from build123d import *

# Parameters (mm, degrees)
F1_DEPTH        = 25
F2_DEPTH        = 30
F3_W            = 11.9576826692
F3_H            = 39.7608936764
F4_DEPTH        = 40
F5_R            = 15.1725757167
F6_DEPTH        = 68.3238299022
F7_T1_DEPTH     = 111.9576826692
F7_T3_DEPTH     = 111.9576826692
F8_R            = 9
F10_D           = 8
F10_DEPTH       = 10
F10_CBORE_D     = 10
F10_CBORE_DEPTH = 5
F10_TIP         = 2.4034424761


# Not quite as in the source:
# - a fillet or chamfer that OpenCascade refuses, or shapes differently, is made with other operations: its cross-section is extruded or revolved along the edge and cut away or added


with BuildPart() as f1:
    # F0 (on Top) → F1 (new body)
    with BuildSketch(Plane.XY):
        with BuildLine():
            Line((8.5056748986, -46.3761053979), (13.5056748986, -46.3761053979))
            Line((13.5056748986, -46.3761053979), (13.5056748986, -23.932851851))
            ThreePointArc((13.5056748986, -23.932851851), (0, -10.4271769524), (-13.5056748986, -23.932851851))
            Line((-13.5056748986, -23.932851851), (-13.5056748986, -46.3761053979))
            Line((-13.5056748986, -46.3761053979), (-8.5056748986, -46.3761053979))
            Line((-8.5056748986, -46.3761053979), (-8.5056748986, -23.932851851))
            ThreePointArc((-8.5056748986, -23.932851851), (0, -15.4271769524), (8.5056748986, -23.932851851))
            Line((8.5056748986, -23.932851851), (8.5056748986, -46.3761053979))
        make_face()
    extrude(amount=F1_DEPTH)

    # F0 (on Top) → F2 (join)
    with BuildSketch(Plane.XY):
        with BuildLine():
            Line((34.1614149511, -46.3761053979), (34.1614149511, 46.3761053979))
            Line((34.1614149511, 46.3761053979), (-34.1614149511, 46.3761053979))
            Line((-34.1614149511, 46.3761053979), (-34.1614149511, -46.3761053979))
            Line((-34.1614149511, -46.3761053979), (-13.5056748986, -46.3761053979))
            Line((-13.5056748986, -46.3761053979), (-13.5056748986, -23.932851851))
            ThreePointArc((-13.5056748986, -23.932851851), (0, -10.4271769524), (13.5056748986, -23.932851851))
            Line((13.5056748986, -23.932851851), (13.5056748986, -46.3761053979))
            Line((13.5056748986, -46.3761053979), (34.1614149511, -46.3761053979))
        make_face()
    extrude(amount=F2_DEPTH)

    # F3 (on face) → F4 (join)
    with BuildSketch(Plane.XY.offset(30)):
        with Locations((28.1825736165, 26.4956585597)):
            Rectangle(F3_W, F3_H)
        with Locations((-28.1825736165, 26.4956585597)):
            Rectangle(F3_W, F3_H)
    extrude(amount=F4_DEPTH)

    # F5 (on face) → F6 (cut, through all)
    with BuildSketch(Plane(origin=(-34.1614149511, 0, 0), x_dir=(0, -1, 0), z_dir=(-1, 0, 0))):
        with Locations((-26.4956585597, 50)):
            Circle(F5_R)
    extrude(amount=-F6_DEPTH, mode=Mode.SUBTRACT)

    # F7: fillet of radius 20 on 4 edges, made by hand

    # F7_s2 → F7_t1 (cut)
    with BuildSketch(Plane.YZ.offset(-84.1614149511)):
        with BuildLine():
            ThreePointArc((6.6152117215, 50), (12.4730760978, 64.1421356237), (26.6152117215, 70))
            Line((26.6152117215, 70), (6.6152117215, 70))
            Line((6.6152117215, 70), (6.6152117215, 50))
        make_face()
        with BuildLine():
            ThreePointArc((46.3761053979, 50), (40.5182410217, 64.1421356237), (26.3761053979, 70))
            Line((26.3761053979, 70), (46.3761053979, 70))
            Line((46.3761053979, 70), (46.3761053979, 50))
        make_face()
    extrude(amount=F7_T1_DEPTH, mode=Mode.SUBTRACT)

    # F7_s4 → F7_t3 (cut)
    with BuildSketch(Plane.YZ.offset(-27.7962677181)):
        with BuildLine():
            ThreePointArc((6.6152117215, 50), (12.4730760978, 64.1421356237), (26.6152117215, 70))
            Line((26.6152117215, 70), (6.6152117215, 70))
            Line((6.6152117215, 70), (6.6152117215, 50))
        make_face()
        with BuildLine():
            ThreePointArc((46.3761053979, 50), (40.5182410217, 64.1421356237), (26.3761053979, 70))
            Line((26.3761053979, 70), (46.3761053979, 70))
            Line((46.3761053979, 70), (46.3761053979, 50))
        make_face()
    extrude(amount=F7_T3_DEPTH, mode=Mode.SUBTRACT)

    # F8
    f8_edges = [f1.edges().sort_by_distance(p)[0] for p in [
        (34.161415, -46.376105, 15),
        (-34.161415, -46.376105, 15),
    ]]
    fillet(f8_edges, radius=F8_R)

    # F10
    with Locations(Plane.XY.offset(30)):
        with Locations((0, 26.4956585597)):
            CounterBoreHole(F10_D / 2, F10_CBORE_D / 2, F10_CBORE_DEPTH, depth=F10_DEPTH)
            with Locations((0, 0, -(F10_DEPTH + F10_TIP / 2))):  # 118° drill point
                Cone(0, F10_D / 2, F10_TIP, mode=Mode.SUBTRACT)


solid = f1.part
Input: part model. Units: mm. Frame: model coordinates. A direction names the side the tool comes from. Give positions to 0.01 mm unless a question says otherwise; leave off trailing zeros. Order: outer loops, then holes, each group sorted by start corner. A loop starts at its lowest first (then second) coordinate and runs counter-clockwise, first axis right, second up.
Q1. Draft query along X for faces 1 (the cylindrical face through (-31.455, -43.81, 15.21)), 2 (the flat face through (28, 6.615, 40)), 3 (the cylindrical face through (-0.19, -15.43, 12.32)), 4 (the flat face through (0, 1, 30)). Return one class per face: +X half, -X half, draft (parallel to the pull), parting line (faces both ways), or undercut.
Checked values:
face 1: -X half
face 2: draft
face 3: undercut
face 4: undercut
Q2. Ray query, probe 1 along Y at (x, z) = (0, 27); probe 2 along X at (y, z) = (-36, 23); probe 3 along X at (y, z) = (9, 55.5). Return the intervals inside material, ascending.
Checked values:
probe 1: y = -10.43 to 21.5, 31.5 to 46.38
probe 2: x = -34.16 to -8.51, 8.51 to 34.16
probe 3: x = -34.16 to -22.2, 22.2 to 34.16
Q3. Section B-B on z = 36. Output: boundary loops of the cut face in (x, y).
Checked values:
outline: (-34.16, 6.62) - (-22.2, 6.62) - (-22.2, 20.65) - (-34.16, 20.65) - close; (-34.16, 32.34) - (-22.2, 32.34) - (-22.2, 46.38) - (-34.16, 46.38) - close; (22.2, 6.62) - (34.16, 6.62) - (34.16, 20.65) - (22.2, 20.65) - close; (22.2, 32.34) - (34.16, 32.34) - (34.16, 46.38) - (22.2, 46.38) - close
Q4. Contact query for flat-ended pins moving along their axis: pin 1 Ø21.5 at (x, y) = (-2, -28) entering from +Z; pin 2 Ø13 at (x, z) = (-28.5, 43) entering from -Y; pin 3 Ø1.5 at (x, y) = (11, 35) entering from +Z. Output: stop coordinate, or through.
Checked values:
pin 1: stops at z = 25
pin 2: stops at y = 6.62
pin 3: stops at z = 30
Q5. Set-up query: faces 5 (the flat face through (-4, 25, 25)), 6 (the flat face through (8.506, -35, 12)), 7 (the flat face through (-13.506, -35, 27)), 8 (the flat face through (22.204, 35, 36)). Return all of +Z, -Z, +X, -X, +Y, -Y with unobstructed straight access to the full face (end or side cutting, diameter ignored); none if empty.
Checked values:
face 5: +Z
face 6: +Z, -Z, -Y
face 7: +Z, -Y
face 8: +Z, +Y, -Y
Q6. Section C-C on x = 26.5. Output: boundary loops of the cut face in (y, z).
Checked values:
outline: (-46.28, 0) - (46.38, 0) - (46.38, 50) arc R20 ccw to (26.5, 70) arc R20 ccw to (6.62, 50) - (6.62, 30) - (-46.28, 30) - close; hole circle Ø30.35 at (26.5, 50)
Q7. Section D-D on z = 16.5. Output: boundary loops of the cut face in (x, y), and give its area (3 significant figures).
Checked values:
outline: (-34.16, -37.38) arc R9 ccw to (-25.16, -46.38) - (-8.51, -46.38) - (-8.51, -23.93) arc R8.51 cw to (8.51, -23.93) - (8.51, -46.38) - (25.16, -46.38) arc R9 ccw to (34.16, -37.38) - (34.16, 46.38) - (-34.16, 46.38) - close
area: 5,810 mm2
Q8. Section A-A on y = -29. Output: boundary loops of the cut face in (x, z).
Checked values:
outline: (-34.16, 0) - (-8.51, 0) - (-8.51, 25) - (-13.51, 25) - (-13.51, 30) - (-34.16, 30) - close; (8.51, 0) - (34.16, 0) - (34.16, 30) - (13.51, 30) - (13.51, 25) - (8.51, 25) - close
